from build123d import *

# Parameters (mm, degrees)
SKETCH_2_W      = 45.704303388
SKETCH_2_H      = 23.283324367
SKETCH_2_R      = 1.5
EXTRUDE_1_DEPTH = 0.5


with BuildPart() as part:
    # Эскиз2 → Бобышка-Вытянуть1 (new body)
    with BuildSketch(Plane(origin=(0, 0, 0), x_dir=(1, 0, 0), z_dir=(0, 1, 0))):
        Polygon((113, 129), (102, 129), (99, 124), (91, 124), (91, 129), (80, 129), (80, 124), (0, 124), (0, 0), (124, 0), (124, 124), (113, 124), align=None)
        with Locations((63.748070218, 82.395863996)):
            Rectangle(SKETCH_2_W, SKETCH_2_H, mode=Mode.SUBTRACT)
        with Locations((120, 120)):
            Circle(SKETCH_2_R, mode=Mode.SUBTRACT)
        with Locations((4, 4)):
            Circle(SKETCH_2_R, mode=Mode.SUBTRACT)
        with Locations((120, 4)):
            Circle(SKETCH_2_R, mode=Mode.SUBTRACT)
        with Locations((4, 120)):
            Circle(SKETCH_2_R, mode=Mode.SUBTRACT)
    extrude(amount=EXTRUDE_1_DEPTH)


solid = part.part
The model under review builds one solid part; all positions refer to its coordinate system, in mm. A direction names the side the tool comes from. Round coordinates to 2 decimals unless told otherwise and drop trailing zeros. Loops run counter-clockwise (first coordinate to the right, second up) from the corner with the lowest first, then second, coordinate; pieces in that order, holes last. Notation, with made-up numbers: M 20.5,15.25 L 56.5,15.25 A24 ccw 56.5,49.25 Z; hole C 10,49 d8. An arc over 180 degrees is marked long. Answer as a JSON object with one key per item and string values.
Item 1: We need section C-C, the plane y = 0.4. State the section outline as (x, z) points.
Check sheet entries:
{"outline": "M 0,-124 L 80,-124 L 80,-129 L 91,-129 L 91,-124 L 99,-124 L 102,-129 L 113,-129 L 113,-124 L 124,-124 L 124,0 L 0,0 Z; hole C 4,-120 d3; hole C 4,-4 d3; hole M 40.9,-94.04 L 86.6,-94.04 L 86.6,-70.75 L 40.9,-70.75 Z; hole C 120,-120 d3; hole C 120,-4 d3"}
Item 2: We need section D-D, the plane z = -82. State the section outline as (x, y) points.
Check sheet entries:
{"outline": "M 0,0 L 40.9,0 L 40.9,0.5 L 0,0.5 Z; M 86.6,0 L 124,0 L 124,0.5 L 86.6,0.5 Z"}
Item 3: We need section A-A, the plane z = -120. State the section outline as (x, y) points, and give its area (3 significant figures).
Check sheet entries:
{"outline": "M 0,0 L 2.5,0 L 2.5,0.5 L 0,0.5 Z; M 5.5,0 L 118.5,0 L 118.5,0.5 L 5.5,0.5 Z; M 121.5,0 L 124,0 L 124,0.5 L 121.5,0.5 Z", "area": "59.0 mm2"}
Item 4: Tool access review of faces 1 (the face through (100.5, 0.2, -126.5)), 2 (the face through (61, 0, -65)): name each direction out of +Z, -Z, +X, -X, +Y, -Y from which nothing blocks a thin tool from reaching the whole face with its end or side.
Check sheet entries:
{"face 1": "-Z, +Y, -Y", "face 2": "+Z, -Z, +X, -X, -Y"}
Item 5: We need section B-B, the plane x = 72. State the section outline as (y, z) points, and give its area (3 significant figures).
Check sheet entries:
{"outline": "M 0,-124 L 0.5,-124 L 0.5,-94.04 L 0,-94.04 Z; M 0,-70.75 L 0.5,-70.75 L 0.5,0 L 0,0 Z", "area": "50.4 mm2"}
Item 6: For line 1 along X through (y, z) = (0.2, -4); line 2 along Z through (x, y) = (120, 0.3); line 3 along X through (y, z) = (0.1, -74), list the stretches that pass through material, from the lowest coordinate up.
Check sheet entries:
{"line 1": "0 to 2.5, 5.5 to 118.5, 121.5 to 124", "line 2": "-124 to -121.5, -118.5 to -5.5, -2.5 to 0", "line 3": "0 to 40.9, 86.6 to 124"}
Item 7: The part is to be moulded in two halves that separate along X. For faces 3 (the face through (118.89, 0.25, -121.01)), 4 (the face through (3.805, 0.246, -121.487)), 5 (the face through (61, 0.5, -65)), say which applies: +X half, -X half, draft (parallel to the pull), parting line (faces both ways), or undercut.
Check sheet entries:
{"face 3": "undercut", "face 4": "undercut", "face 5": "draft"}
Item 8: Clearance check with flat-ended pins moving along their axes: P1, Ø4, axis at x = 120, z = -4, coming from the +Y side; P2, Ø2.5, axis at x = 4, z = -4, coming from the -Y side. State where each tip first meets the part, or that it passes through.
Check sheet entries:
{"P1": "y = 0.5", "P2": "through"}
